Autodesk Inventor part; units mm, degrees
ref_plane "Work Plane1" through (0, 0, 5) normal (0, 0, 1) x (1, 0, 0)
ref_plane "YZ Plane" through (0, 0, 0) normal (1, 0, 0) x (0, 1, 0)
ref_plane "XZ Plane" through (0, 0, 0) normal (0, 1, 0) x (-1, 0, 0)
sketch "Sketch1" plane through (0, 0, 0) normal (0, 0, 1) x (1, 0, 0)
  circle A0 centre (0, 0) radius 5.75
  dimension "d0" = 11.5
extrude "Extrusion1" add sketch "Sketch1" along normal blind 7
ref_plane "Work Plane1" through (0, 0, 5) normal (0, 0, 1) x (1, 0, 0)
sketch "Sketch2" plane through (0, 0, 5) normal (0, 0, 1) x (1, 0, 0)
  circle A0 centre (0, 0) radius 5.75
  circle A1 centre (0, 0) radius 5.75
  line L0 (-0.75, 5.7009) -> (-0.75, 6.7009)
  line L1 (-0.75, 6.7009) -> (0.75, 6.7009)
  line L2 (0.75, 6.7009) -> (0.75, 5.7009)
  dimension "d4" = 1.5
  dimension "d5" = 1
extrude "Extrusion2" add sketch "Sketch2" along normal mid plane 0.2 contours A0 L0 L1 L2
pattern_circular "Circular Pattern1" count 12 over 360 about axis through (0, 0, 0) along (0, 0, 1) of "Extrusion2"
sketch "Sketch3" plane through (0, 0, 7) normal (0, 0, 1) x (1, 0, 0)
  circle A0 centre (0, 0) radius 5.75
hole "Hole1" at (0, 0, 7) direction (0, 0, -1) diameter 4 end through all
properties part number "ExtruderCouplingBowden" material "ABS Plastic"
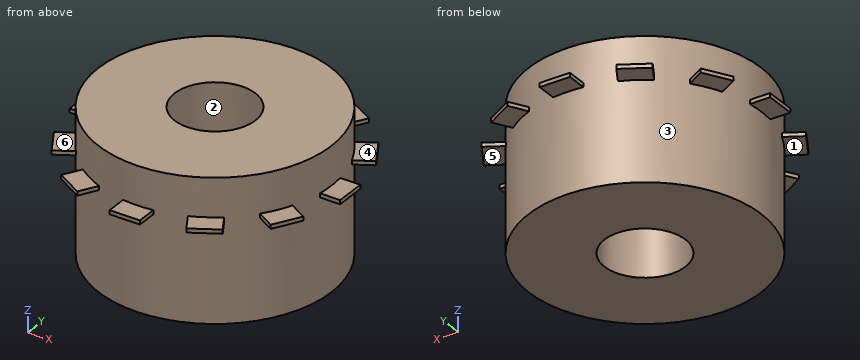
Design review of the part built by this model. Coordinates are the model's own, in mm. Face numbers are marked on the shaded views. A direction names the side the tool comes from. Round coordinates to 2 decimals unless told otherwise and drop trailing zeros. Write each loop counter-clockwise with the first axis right and the second up, starting at its lowest first coordinate (ties: lowest second). Pieces come first, ordered by that corner, then holes. Notation, with made-up numbers: M -5,-32.5 L 23,-32.5 A16 ccw 23,-12.5 Z; hole C -28.5,-26 d2. An arc over 180 degrees is marked long. One line per item, written item: value. Start each with the question number.
1. Take a section at A-A on x = 0. State the section outline as (y, z) points.
2. Take a section at D-D on y = -3. State the section outline as (x, z) points, then the cut area to 3 significant figures.
3. For the marked faces 3, 4, 5 and 6, list the 3-axis set-ups (+Z, -Z, +X, -X, +Y, -Y) from which the entire face can be reached by the end or side of a thin tool; tool diameter is ignored.
4. To check wall thickness, follow probe 1 along X at (y, z) = (0, 4.5); probe 2 along Y at (x, z) = (0, 5). State the ranges of each line that lie inside material, in increasing order. Write a range as from..to.
5. Draft analysis for pull direction Y (two halves, no side actions). For the marked faces 1 and 2, state which applies: pulls with the +Y half, pulls with the -Y half, needs draft (parallel to the pull), parting line crosses it, or undercut.
6. Take a section at C-C on z = 6.5. State the section outline as (x, y) points.
7. Clearance check with flat-ended pins moving along their axes: P1, Ø1.5, axis at y = 2, z = 1, coming from the -X side; P2, Ø2.5, axis at x = 0, y = 0, coming from the -Z side; P3, Ø1, axis at x = -3.5, z = 3.5, coming from the -Y side; P4, Ø0.8, axis at x = 5.5, y = 3.5, coming from the +Z side. State where each tip first meets the part, or that it passes through.
Computed:
1. outline: M -6.7,4.9 L -5.75,4.9 L -5.75,0 L -2,0 L -2,7 L -5.75,7 L -5.75,5.1 L -6.7,5.1 Z; M 2,0 L 5.75,0 L 5.75,4.9 L 6.7,4.9 L 6.7,5.1 L 5.75,5.1 L 5.75,7 L 2,7 Z
2. outline: M -6.01,4.9 L -4.91,4.9 L -4.91,0 L 4.91,0 L 4.91,4.9 L 6.01,4.9 L 6.01,5.1 L 4.91,5.1 L 4.91,7 L -4.91,7 L -4.91,5.1 L -6.01,5.1 Z
2. area: 69.1 mm²
3. face 3: none
3. face 4: +Z, +X, +Y
3. face 5: -Z, +X, +Y
3. face 6: +Z, -X, -Y
4. probe 1: x = -5.75..-2, 2..5.75
4. probe 2: y = -6.7..-2, 2..6.7
5. face 1: needs draft
5. face 2: undercut
6. outline: C 0,0 d11.5; hole C 0,0 d4
7. P1: stops at x = -5.61
7. P2: passes through
7. P3: stops at y = -4.91
7. P4: stops at z = 5.1
